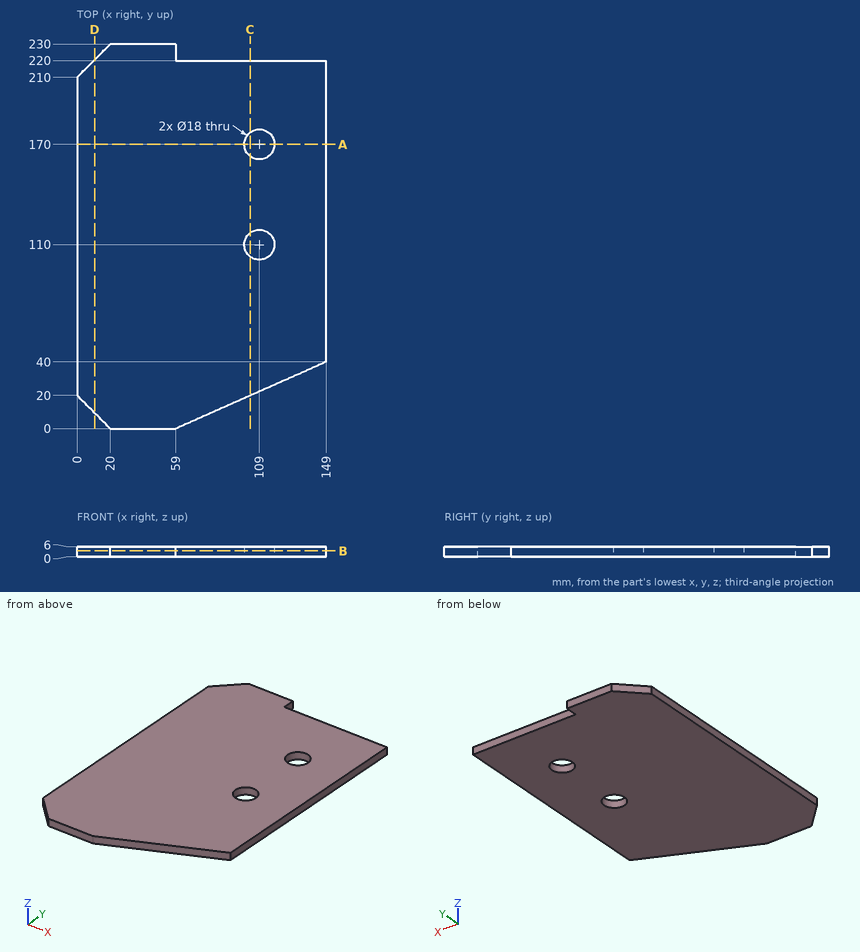
Geometry check sheet. Reference: drawing and pictorial views, mm from the part's lowest x, y, z. Give positions to 0.01 mm unless a question says otherwise; leave off trailing zeros. Loops run counter-clockwise (first coordinate to the right, second up) from the corner with the lowest first, then second, coordinate; pieces in that order, holes last. Notation, with made-up numbers: (84.25, -7) -> (139.25, -7) arc R19 cw to (139.25, 16) -> close; hole circle Ø1 at (4.25, 75.5). An arc over 180 degrees is marked (long way). Answer in a Markdown table with one row per item. Add a question column.
1) Material ranges on probe 1 along Y at (x, z) = (109, 4.3); probe 2 along X at (y, z) = (170, 3.4); probe 3 along X at (y, z) = (177, 1.35), recorded low to high. Write a range as from..to.
2) Cross-section at C-C on x = 103.5. Record the boundary of the cut face in (y, z).
3) Cross-section at D-D on x = 10.5. Record the boundary of the cut face in (y, z).
4) Gauge pin test, flat ends, axial feed: P1, Ø3, axis at x = 108, z = 3, coming from the +Y side; P2, Ø3, axis at x = 116.5, z = 1, coming from the -Y side; P3, Ø1.8, axis at y = 224.5, z = 3, coming from the +X side. Record the tip position at first contact, or that the pin passes through.
5) Cross-section at A-A on y = 170. Record the boundary of the cut face in (x, z), and give its area (3 significant figures).
6) Cross-section at B-B on z = 3.5. Record the boundary of the cut face in (x, y).
Outcome:
| question | item | result |
|---|---|---|
| 1 | probe 1 | y = 22.22..101, 119..161, 179..220 |
| 1 | probe 2 | x = 0..100, 118..149 |
| 1 | probe 3 | x = 0..103.34, 114.66..149 |
| 2 | outline | (19.78, 0) -> (102.88, 0) -> (102.88, 6) -> (19.78, 6) -> close; (117.12, 0) -> (162.88, 0) -> (162.88, 6) -> (117.12, 6) -> close; (177.12, 0) -> (220, 0) -> (220, 6) -> (177.12, 6) -> close |
| 3 | outline | (9.5, 0) -> (220.5, 0) -> (220.5, 6) -> (9.5, 6) -> close |
| 4 | P1 | stops at y = 220 |
| 4 | P2 | stops at y = 24.89 |
| 4 | P3 | stops at x = 59 |
| 5 | outline | (0, 0) -> (100, 0) -> (100, 6) -> (0, 6) -> close; (118, 0) -> (149, 0) -> (149, 6) -> (118, 6) -> close |
| 5 | area | 786 mm^2 |
| 6 | outline | (0, 20) -> (20, 0) -> (59, 0) -> (149, 40) -> (149, 220) -> (59, 220) -> (59, 230) -> (20, 230) -> (0, 210) -> close; hole circle Ø18 at (109, 110); hole circle Ø18 at (109, 170) |
